```python
from build123d import *

# Parameters (mm, degrees)
BOSS_EXTRUDE1_DEPTH = 3.13
SKETCH2_R           = 4.05
CUT_EXTRUDE1_DEPTH  = 3.13
SKETCH3_R           = 1.5
CUT_EXTRUDE2_DEPTH  = 17
SKETCH4_W           = 26.4
SKETCH4_H           = 32.8
BOSS_EXTRUDE2_DEPTH = 3.13
SKETCH5_R           = 4.95
CUT_EXTRUDE3_DEPTH  = 3.13
SKETCH6_R           = 1.75
CUT_EXTRUDE4_DEPTH  = 3.13


with BuildPart() as part:
    # Sketch1 → Boss-Extrude1 (new body)
    with BuildSketch(Plane.XY):
        with BuildLine():
            Line((-13.2, 20.24), (-13.2, 0))
            ThreePointArc((-13.2, 0), (0, 13.2), (13.2, 0))
            Line((13.2, 0), (13.2, 20.24))
            Line((13.2, 20.24), (-13.2, 20.24))
        make_face()
        with BuildLine():
            Line((-13.2, 0), (0, 0))
            Line((0, 0), (13.2, 0))
            ThreePointArc((13.2, 0), (0, 13.2), (-13.2, 0))
        make_face()
        with BuildLine():
            Line((13.2, 0), (0, 0))
            Line((0, 0), (0, -13.2))
            ThreePointArc((0, -13.2), (9.333809512, -9.333809512), (13.2, 0))
        make_face()
        with BuildLine():
            Line((0, -13.2), (0, 0))
            Line((0, 0), (-13.2, 0))
            ThreePointArc((-13.2, 0), (-9.333809512, -9.333809512), (0, -13.2))
        make_face()
    extrude(amount=-BOSS_EXTRUDE1_DEPTH)

    # Sketch2 → Cut-Extrude1 (cut)
    with BuildSketch(Plane.XY):
        Circle(SKETCH2_R)
    extrude(amount=-CUT_EXTRUDE1_DEPTH, mode=Mode.SUBTRACT)

    # Sketch3 → Cut-Extrude2 (cut)
    with BuildSketch(Plane.XY):
        with Locations((8.5, 0)):
            Circle(SKETCH3_R)
        with Locations((-8.5, 0)):
            Circle(SKETCH3_R)
    extrude(amount=-CUT_EXTRUDE2_DEPTH, mode=Mode.SUBTRACT)

    # Sketch4 → Boss-Extrude2 (add)
    with BuildSketch(Plane(origin=(0, 20.24, 0), x_dir=(1, 0, 0), z_dir=(0, 1, 0))):
        with Locations((0, 16.4)):
            Rectangle(SKETCH4_W, SKETCH4_H)
    extrude(amount=-BOSS_EXTRUDE2_DEPTH)

    # Sketch5 → Cut-Extrude3 (cut)
    with BuildSketch(Plane(origin=(0, 20.24, 0), x_dir=(1, 0, 0), z_dir=(0, 1, 0))):
        with Locations(Location((0, 16.4, 0), (0, 0, 270))):
            Circle(SKETCH5_R)
    extrude(amount=-CUT_EXTRUDE3_DEPTH, mode=Mode.SUBTRACT)

    # Sketch6 → Cut-Extrude4 (cut)
    with BuildSketch(Plane(origin=(0, 20.24, 0), x_dir=(1, 0, 0), z_dir=(0, 1, 0))):
        with Locations(Location((8, 23.4, 0), (0, 0, 270))):
            Circle(SKETCH6_R)
        with Locations(Location((8, 9.4, 0), (0, 0, 270))):
            Circle(SKETCH6_R)
        with Locations(Location((-8, 9.4, 0), (0, 0, 270))):
            Circle(SKETCH6_R)
        with Locations(Location((-8, 23.4, 0), (0, 0, 270))):
            Circle(SKETCH6_R)
    extrude(amount=-CUT_EXTRUDE4_DEPTH, mode=Mode.SUBTRACT)


solid = part.part
```
Work out the finished part from the listing and answer in its coordinate system (mm). A direction names the side the tool comes from. Round coordinates to 2 decimals unless told otherwise and drop trailing zeros. Write each loop counter-clockwise with the first axis right and the second up, starting at its lowest first coordinate (ties: lowest second). Pieces come first, ordered by that corner, then holes.
1) A cutting plane is placed at D-D on x = 8. Determine the outline of the cut face in (y, z).
2) Which of the six approach directions +Z, -Z, +X, -X, +Y, -Y give full straight-line access (tool end or side, diameter ignored) to faces 4 (the face through (-13.2, 18, -11)), 5 (the face through (-0.2, 17.11, -21.5))?
3) A cutting plane is placed at B-B on z = -2. Determine the outline of the cut face in (x, y).
4) Determine the mould class of faces 1 (the face through (7.3, -0.9, -1.5)), 2 (the face through (0, 19, -32.8)), 3 (the face through (1.49, 18.7, -11.68)) for opening direction Z: pulls with the +Z half, pulls with the -Z half, needs draft (parallel to the pull), parting line crosses it, or undercut.
5) Consider probe 1 along X at (y, z) = (18.55, -16.4); probe 2 along Z at (x, y) = (2.5, 13); probe 3 along Y at (x, z) = (5, -26). Determine where each line is inside the solid, lowest interval first.
6) A cutting plane is placed at C-C on x = -2.5. Determine the outline of the cut face in (y, z), and give its area (3 significant figures).
7) Flat-ended cylindrical pins translate along their axes: P1, Ø4, axis at x = 8.5, y = 0, coming from the -Z side; P2, Ø5.5, axis at x = -8, z = -23.4, coming from the -Y side; P3, Ø6, axis at y = -9, z = -4.5, coming from the +X side. Find the tip coordinate at first contact, or state that the pin passes through.
8) A cutting plane is placed at A-A on z = -9.4. Determine the outline of the cut face in (x, y), and give its area (3 significant figures).
Entries:
1. outline: (-10.5, -3.13) - (-1.41, -3.13) - (-1.41, 0) - (-10.5, 0) - close; (1.41, -3.13) - (17.11, -3.13) - (17.11, -7.65) - (20.24, -7.65) - (20.24, 0) - (1.41, 0) - close; (17.11, -32.8) - (20.24, -32.8) - (20.24, -25.15) - (17.11, -25.15) - close; (17.11, -21.65) - (20.24, -21.65) - (20.24, -11.15) - (17.11, -11.15) - close
2. face 4: +Z, -Z, -X, +Y, -Y
2. face 5: -Z, +X, -X, -Y
3. outline: (-13.2, 0) arc R13.2 ccw to (13.2, 0) - (13.2, 20.24) - (-13.2, 20.24) - close; hole circle Ø3 at (-8.5, 0); hole circle Ø8.1 at (0, 0); hole circle Ø3 at (8.5, 0)
4. face 1: needs draft
4. face 2: pulls with the -Z half
4. face 3: undercut
5. probe 1: x = -13.2 to -4.95, 4.95 to 13.2
5. probe 2: z = -3.13 to 0
5. probe 3: y = 17.11 to 20.24
6. outline: (-12.96, -3.13) - (-3.19, -3.13) - (-3.19, 0) - (-12.96, 0) - close; (3.19, -3.13) - (17.11, -3.13) - (17.11, -12.13) - (20.24, -12.13) - (20.24, 0) - (3.19, 0) - close; (17.11, -32.8) - (20.24, -32.8) - (20.24, -20.67) - (17.11, -20.67) - close
6. area: 150 mm2
7. P1: stops at z = -3.13
7. P2: stops at y = 17.11
7. P3: stops at x = 11.58
8. outline: (-13.2, 17.11) - (-9.75, 17.11) - (-9.75, 20.24) - (-13.2, 20.24) - close; (-6.25, 17.11) - (6.25, 17.11) - (6.25, 20.24) - (-6.25, 20.24) - close; (9.75, 17.11) - (13.2, 17.11) - (13.2, 20.24) - (9.75, 20.24) - close
8. area: 60.7 mm2
